Build history of the part. All positions in model axes, mm. Give positions to 0.01 mm unless a question says otherwise; leave off trailing zeros. Order: outer loops, then holes, each group sorted by start corner. A loop starts at its lowest first (then second) coordinate and runs counter-clockwise, first axis right, second up. Notation, with made-up numbers: (-27, -33.5) - (-18, -33.5) arc R13 cw to (-18, -17.5) - close; hole circle Ø8 at (85, 26). An arc over 180 degrees is marked (long way). Use a Markdown table: item, result. Add a question column.
(1) Slice it at B-B (x = 3.5). Write the cut outline in (y, z) (1 decimal).
(2) Flat gauge pins, fed straight in: pin 1 (4 mm diameter, centred on x = 4.5, z = 5.5, fed in from +Y); pin 2 (1.5 mm diameter, centred on x = 6, y = -6.5, fed in from -Z). Where does each tip first touch, or does it go through?
(3) Wall check: line 1 (Z direction, x = 3, y = 0); line 2 (Z direction, x = 6.5, y = 2.75); line 3 (Y direction, x = 4.5, z = 1.5). Give the ranges that are in metal, low to high.
(4) Mould opens along Y. For faces 1 (the face through (4, 0, -8.5)), 2 (the face through (3.951, -7.396, 4.19)), 3 (the face through (3.951, 7.327, 4.31)), 4 (the face through (3.95, 2.63, 3.43)) say: +Y half, -Y half, draft (parallel to the pull), parting line (faces both ways), or undercut.
(5) Slice it at A-A (y = 0). Write the cut outline in (x, z), then the cut area to 3 significant figures.
Autodesk Inventor part; units mm, degrees
ref_plane "Work Plane1" through (-19.2723, 0, 0) normal (0, -0.866, -0.5) x (1, 0, 0)
ref_plane "YZ Plane" through (0, 0, 0) normal (1, 0, 0) x (0, 1, 0)
ref_plane "XZ Plane" through (0, 0, 0) normal (0, 1, 0) x (-1, 0, 0)
sketch "Sketch1" plane through (0, 0, 0) normal (1, 0, 0) x (0, 1, 0)
  line L0 (-9.815, 0) -> (-4.9075, 8.5)
  line L1 (-4.9075, 8.5) -> (4.9075, 8.5)
  line L2 (4.9075, 8.5) -> (9.815, 0)
  line L3 (9.815, 0) -> (4.9075, -8.5)
  line L4 (4.9075, -8.5) -> (-4.9075, -8.5)
  line L5 (-4.9075, -8.5) -> (-9.815, 0)
  point P0 (0, 0)
  point P1 (0, 0)
  dimension "d0" = 19.6299
extrude "Body" add sketch "Sketch1" along normal blind 8
sketch "Sketch2" plane through (0, 0, 0) normal (0, 0, 1) x (1, 0, 0)
  line L0 (0, 4.9075) -> (0, 9.815)
  line L1 (0, 9.815) -> (8, 9.815)
  line L2 (8, 4.9075) -> (8, 9.815)
  line L3 (-1.6, 0) -> (9.6, 0)
  line L4 (1.2499, 9.815) -> (0, 7.65)
  line L5 (6.7501, 9.815) -> (8, 7.65)
  dimension "d3" = 30
  dimension "d4" = 30
  dimension "d5" = 15.3
  dimension "d6" = 15.3
revolve "Chamfer1" cut sketch "Sketch2" angle 360 about axis through (-10, 0, 0) along (1, 0, 0)
sketch "Sketch3" plane through (8, 0, 0) normal (1, 0, 0) x (0, 0, -1)
  arc A0 (-0.625, -1.0825) -> (0.625, -1.0825) centre (0, 0) ccw
hole "Thread" at (8, 0, 0) direction (-1, 0, 0) diameter 8.647 end through all
chamfer "Chamfer2" distance 0.6766 angle 30 1 edges at (8, 0, 4.3235) measured on face at (8, 6.4566, -0.784)
chamfer "Chamfer3" distance 0.6766 angle 30 1 edges at (0, 0, 4.3235) measured on face at (0, 6.4566, -0.784)
ref_plane "Work Plane1" through (-19.2723, 0, 0) normal (0, -0.866, -0.5) x (1, 0, 0)
equation "\"d0\" = 1.1547 * SW"
equation "\"d1\" = KOH"
equation "\"d8\" = -0.5 * GD1 + 0.5 * NND"
equation "\"d40\" = -0.5 * GD1 + 0.5 * NND"
equation "\"d10\" = -0.5 * GD1 + 0.5 * NND"
equation "\"d41\" = -0.5 * GD1 + 0.5 * NND"
equation "\"d3\" = ANG1"
equation "\"d4\" = ANG2"
equation "\"d5\" = SW0"
equation "\"d6\" = SW01"
equation "\"ANG1\" = 30deg"
equation "\"ANG2\" = 30deg"
equation "\"KOH\" = 8"
equation "\"SW\" = 17"
equation "\"SW0\" = SW01"
equation "\"SW01\" = 15.3"
equation "\"GUL\" = 0.541266 * PTC"
equation "\"TOA\" = 30deg"
equation "\"PTC\" = 1.25"
equation "\"E0\" = 1.155 * SW"
equation "\"GAL\" = 0.541266 * PTC"
properties part number "DIN 934 - M10 x 1,25" material "Steel, Mild"
Solution:
| question | item | result |
|---|---|---|
| 1 | outline | (-9.8, 0) - (-4.9, -8.5) - (4.9, -8.5) - (9.8, 0) - (4.9, 8.5) - (-4.9, 8.5) - close; hole circle Ø8.6 at (0, 0) |
| 2 | pin 1 | y = 7.79 |
| 2 | pin 2 | z = -7.04 |
| 3 | line 1 | -8.5 to -4.32, 4.32 to 8.5 |
| 3 | line 2 | -8.5 to -3.34, 3.34 to 8.5 |
| 3 | line 3 | -8.95 to -4.05, 4.05 to 8.95 |
| 4 | face 1 | draft |
| 4 | face 2 | -Y half |
| 4 | face 3 | +Y half |
| 4 | face 4 | undercut |
| 5 | outline | (0, -7.65) - (0.49, -8.5) - (7.51, -8.5) - (8, -7.65) - (8, -5) - (7.61, -4.32) - (0.39, -4.32) - (0, -5) - close; (0, 5) - (0.39, 4.32) - (7.61, 4.32) - (8, 5) - (8, 7.65) - (7.51, 8.5) - (0.49, 8.5) - (0, 7.65) - close |
| 5 | area | 65.5 mm2 |
